The listing builds one solid part. Answer for the finished solid, in the listing's coordinates (mm). Face numbers are marked on the shaded views. Round coordinates to 2 decimals unless told otherwise and drop trailing zeros. Write each loop counter-clockwise with the first axis right and the second up, starting at its lowest first coordinate (ties: lowest second). Pieces come first, ordered by that corner, then holes. Notation, with made-up numbers: M 15.25,-4 L 24.25,-4 A22 cw 24.25,13 Z; hole C 22,-21 d10. An arc over 180 degrees is marked long. Write each question's results on one line, items separated by ' | '.
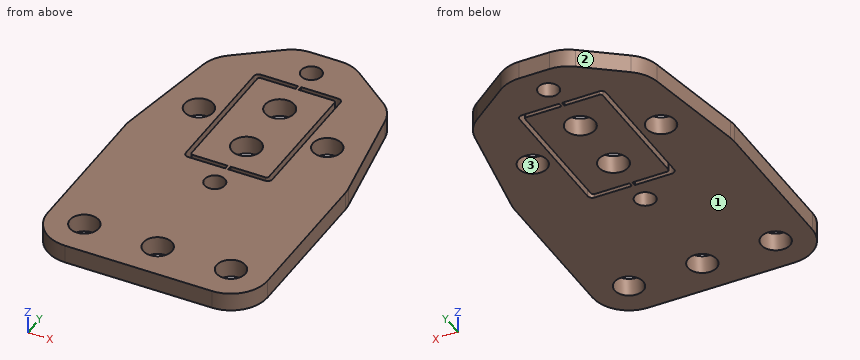
Autodesk Inventor part; units mm, degrees
ref_plane "YZ Plane" through (0, 0, 0) normal (1, 0, 0) x (0, 1, 0)
ref_plane "XZ Plane" through (0, 0, 0) normal (0, 1, 0) x (-1, 0, 0)
ref_plane "XY Plane" through (0, 0, 0) normal (0, 0, 1) x (1, 0, 0)
sketch "Sketch1" plane through (0, 0, 0) normal (0, 0, 1) x (1, 0, 0)
  line L0 (19.05, 12.7) -> (-19.05, 12.7)
  line L1 (-19.05, 12.7) -> (-19.05, -12.7)
  line L2 (-19.05, -12.7) -> (19.05, -12.7)
  line L3 (19.05, -12.7) -> (19.05, 12.7)
  circle A0 centre (-12.7, 0) radius 2.4892
  line L4 (-12.7, 0) -> (12.7, 0)
  circle A1 centre (12.7, 0) radius 2.4892
  line L5 (-19.05, -6.35) -> (19.05, -6.35)
  circle A2 centre (-11.1125, 34.925) radius 2.4892
  line L6 (-11.1125, 34.925) -> (11.1125, 34.925)
  circle A3 centre (11.1125, 34.925) radius 2.4892
  line L7 (-19.05, 12.7) -> (-19.05, 26.343)
  line L8 (-19.05, 26.343) -> (-15.3495, 47.625)
  line L9 (-15.3495, 47.625) -> (15.3495, 47.625)
  line L10 (15.3495, 47.625) -> (19.05, 26.343)
  line L11 (19.05, 26.343) -> (19.05, 12.7)
  circle A4 centre (-11.1125, 34.925) radius 6.35 construction
  circle A5 centre (0, 29.425) radius 2.54
  circle A6 centre (0, 40.425) radius 2.54
  line L12 (0, 40.425) -> (0, 29.425)
  circle A7 centre (0, 0) radius 2.4892
  line L13 (7.493, 46.99) -> (-7.493, 46.99)
  line L14 (-7.493, 46.99) -> (-7.493, 22.86)
  line L15 (-7.493, 22.86) -> (7.493, 22.86)
  line L16 (7.493, 22.86) -> (7.493, 46.99)
  line L17 (7.493, 46.99) -> (-7.493, 22.86) construction
  line L18 (-7.493, 46.99) -> (7.493, 22.86) construction
  circle A8 centre (0, 50.925) radius 1.778
  circle A9 centre (0, 18.925) radius 1.778
  line L19 (-15.3495, 47.625) -> (-4.7625, 55.6875)
  line L20 (4.7625, 55.6875) -> (15.3495, 47.625)
  line L21 (-7.493, 34.925) -> (7.493, 34.925) construction
  line L22 (-7.493, 37.3062) -> (7.493, 37.3062)
  line L23 (-7.493, 34.1313) -> (7.493, 34.1313)
  line L24 (4.7625, 55.6875) -> (-4.7625, 55.6875)
  line L25 (7.493, 37.3062) -> (7.493, 34.1313)
  line L26 (-7.493, 37.3062) -> (-7.493, 34.1313)
  line L27 (-6.6992, 46.1963) -> (6.6992, 46.1963)
  line L28 (6.6992, 46.1963) -> (6.6992, 23.6537)
  line L29 (6.6992, 23.6537) -> (-6.6992, 23.6537)
  line L30 (-6.6992, 23.6537) -> (-6.6992, 46.1963)
  line L31 (0.254, 46.99) -> (-0.254, 46.99)
  line L32 (-0.254, 46.99) -> (-0.254, 46.1963)
  line L33 (-0.254, 46.1963) -> (0.254, 46.1963)
  line L34 (0.254, 46.1963) -> (0.254, 46.99)
  line L35 (0.254, 46.99) -> (-0.254, 46.1963) construction
  line L36 (-0.254, 46.99) -> (0.254, 46.1963) construction
  line L37 (0.254, 22.86) -> (-0.254, 22.86)
  line L38 (-0.254, 22.86) -> (-0.254, 23.6537)
  line L39 (-0.254, 23.6537) -> (0.254, 23.6537)
  line L40 (0.254, 23.6537) -> (0.254, 22.86)
  line L41 (0.254, 22.86) -> (-0.254, 23.6537) construction
  line L42 (-0.254, 22.86) -> (0.254, 23.6537) construction
  point P0 (0, 12.7)
  point P1 (0, 47.625)
  point P2 (0, 34.925)
  point P3 (0, 34.925)
  point P4 (0, 34.925)
  point P5 (-7.493, 34.1313)
  point P6 (7.493, 34.1313)
  point P7 (7.493, 37.3062)
  point P8 (-7.493, 37.3062)
  point P9 (0, 55.6875)
  point P10 (0, -12.7)
  point P11 (0, 46.5931)
  point P12 (0, 46.5931)
  point P13 (0, 23.2569)
  point P14 (0, 23.2569)
  dimension "d0" = 38.1
  dimension "d1" = 25.4
  dimension "d2" = 4.9784
  dimension "d3" = 4.9784
  dimension "d4" = 25.4
  dimension "d5" = 6.35
  dimension "d6" = 4.9784
  dimension "d7" = 22.225
  dimension "d8" = 22.225
  dimension "d9" = 21.282
  dimension "d10" = 12.7
  dimension "d11" = 12.7
  dimension "d12" = 5.08
  dimension "d13" = 11
  dimension "d17" = 24.13
  dimension "d18" = 14.986
  dimension "d19" = 3.556
  dimension "d22" = 360
  dimension "d24" = 32
  dimension "d29" = 0.7937
  dimension "d31" = 3.175
  dimension "d32" = 4.7625
  dimension "d33" = 9.525
  dimension "d51" = 12.7
  dimension "d52" = 6.35
  dimension "d53" = 0.7937
  dimension "d54" = 0.508
extrude "Plate1" add sketch "Sketch1" along normal blind 3.175 contours L3 L5 L1 L0 | L0 L7 L8 L9 L10 L11 | L9 L19 L24 L20 | L30 L22 L12 L6 | L6 L12 L23 L30 | L12 L22 L28 L6 | L6 L28 L23 L12 | L23 L28 L29 L30 | L30 L27 L28 L22 | L13 L34 L27 L32 | L38 L29 L40 L15
fillet "Corner Round2" radius 6.35 8 edges at (19.05, -6.35, 1.5875) (-19.05, -6.35, 1.5875) (19.05, 26.343, 1.5875) (-15.3495, 47.625, 1.5875) (-4.7625, 55.6875, 1.5875) (4.7625, 55.6875, 1.5875) (15.3495, 47.625, 1.5875) (-19.05, 26.343, 1.5875)
cut "Cut1" [suppressed]
fillet "Corner Round3" radius 0.7937 4 edges at (-7.493, 46.99, 1.5875) (-7.493, 22.86, 1.5875) (7.493, 22.86, 1.5875) (7.493, 46.99, 1.5875)
fillet "Corner Round4" radius 0.3969 4 edges at (6.6992, 46.1963, 1.5875) (-6.6992, 46.1963, 1.5875) (-6.6992, 23.6537, 1.5875) (6.6992, 23.6537, 1.5875)
sketch "Sketch4" plane through (0, 0, 3.175) normal (0, 0, 1) x (1, 0, 0)
  line L0 (0.254, 46.99) -> (6.6992, 46.99)
  arc A0 (7.493, 46.1963) -> (6.6992, 46.99) centre (6.6992, 46.1963) ccw
  line L1 (7.493, 46.1963) -> (7.493, 23.6538)
  arc A1 (6.6992, 22.86) -> (7.493, 23.6538) centre (6.6992, 23.6538) ccw
  line L2 (6.6992, 22.86) -> (0.254, 22.86)
  arc A2 (-7.493, 23.6538) -> (-6.6993, 22.86) centre (-6.6993, 23.6538) ccw
  line L3 (-7.493, 23.6538) -> (-7.493, 46.1963)
  arc A3 (-6.6993, 46.99) -> (-7.493, 46.1963) centre (-6.6993, 46.1963) ccw
  arc A4 (-18.9561, 26.8828) -> (-19.05, 25.795) centre (-12.7, 25.795) ccw
  line L4 (-19.05, 0) -> (-19.05, 25.795)
  arc A5 (-19.05, 0) -> (-12.7, -6.35) centre (-12.7, 0) ccw
  line L5 (12.7, -6.35) -> (-12.7, -6.35)
  arc A6 (12.7, -6.35) -> (19.05, 0) centre (12.7, 0) ccw
  line L6 (19.05, 25.795) -> (19.05, 0)
  arc A7 (19.05, 25.795) -> (18.9561, 26.8828) centre (12.7, 25.795) ccw
  line L7 (15.7763, 45.1704) -> (18.9561, 26.8828)
  arc A8 (15.7763, 45.1704) -> (13.3674, 49.1345) centre (9.5202, 44.0826) ccw
  line L8 (6.4671, 54.3894) -> (13.3674, 49.1345)
  arc A9 (6.4671, 54.3894) -> (2.6199, 55.6875) centre (2.6199, 49.3375) ccw
  line L9 (-2.6199, 55.6875) -> (2.6199, 55.6875)
  arc A10 (-2.6199, 55.6875) -> (-6.4671, 54.3894) centre (-2.6199, 49.3375) ccw
  line L10 (-13.3674, 49.1345) -> (-6.4671, 54.3894)
  arc A11 (-13.3674, 49.1345) -> (-15.7763, 45.1704) centre (-9.5202, 44.0826) ccw
  line L11 (-18.9561, 26.8828) -> (-15.7763, 45.1704)
  circle A12 centre (11.1125, 34.925) radius 2.4892
  circle A13 centre (-11.1125, 34.925) radius 2.4892
  circle A14 centre (0, 18.925) radius 1.778
  circle A15 centre (0, 0) radius 2.4892
  circle A16 centre (12.7, 0) radius 2.4892
  circle A17 centre (-12.7, 0) radius 2.4892
  circle A18 centre (0, 50.925) radius 1.778
  line L12 (-27.7407, 9.4742) -> (24.6669, 9.4742)
  arc A19 (-11.4438, 46.6085) -> (-12.6483, 44.6265) centre (-9.5202, 44.0826) ccw
  line L13 (-11.4438, 46.6085) -> (-4.5435, 51.8634)
  arc A20 (-2.6199, 52.5125) -> (-4.5435, 51.8634) centre (-2.6199, 49.3375) ccw
  line L14 (-2.6199, 52.5125) -> (2.6199, 52.5125)
  arc A21 (4.5435, 51.8634) -> (2.6199, 52.5125) centre (2.6199, 49.3375) ccw
  line L15 (4.5435, 51.8634) -> (11.4438, 46.6085)
  arc A22 (12.6483, 44.6265) -> (11.4438, 46.6085) centre (9.5202, 44.0826) ccw
  line L16 (12.6483, 44.6265) -> (15.8281, 26.3389)
  arc A23 (15.875, 25.795) -> (15.8281, 26.3389) centre (12.7, 25.795) ccw
  line L17 (15.875, 25.795) -> (15.875, 0)
  arc A24 (12.7, -3.175) -> (15.875, 0) centre (12.7, 0) ccw
  line L18 (12.7, -3.175) -> (-12.7, -3.175)
  arc A25 (-15.875, 0) -> (-12.7, -3.175) centre (-12.7, 0) ccw
  line L19 (-15.875, 0) -> (-15.875, 25.795)
  arc A26 (-15.8281, 26.3389) -> (-15.875, 25.795) centre (-12.7, 25.795) ccw
  line L20 (-15.8281, 26.3389) -> (-12.6483, 44.6265)
  line L21 (-8.6233, 15.877) -> (8.6233, 15.877)
  line L22 (8.6233, 15.877) -> (15.8281, 26.3389)
  line L23 (-8.6233, 15.877) -> (-15.8281, 26.3389)
  line L24 (-8.6233, 15.877) -> (-8.6233, 5.6134)
  line L25 (-8.6233, 5.6134) -> (-15.875, 5.6134)
  line L26 (8.6233, 15.877) -> (8.6233, 5.6134)
  line L27 (8.6233, 5.6134) -> (15.875, 5.6134)
  line L28 (-10.0711, 17.9793) -> (-10.0711, 5.6134)
  line L29 (10.0711, 17.9793) -> (10.0711, 5.6134)
  arc A27 (6.3024, 23.6537) -> (6.6992, 24.0506) centre (6.3024, 24.0506) ccw
  line L30 (6.6992, 45.7994) -> (6.6992, 24.0506)
  arc A28 (6.6992, 45.7994) -> (6.3024, 46.1963) centre (6.3024, 45.7994) ccw
  line L31 (0.254, 46.1963) -> (6.3024, 46.1963)
  line L32 (0.254, 46.99) -> (0.254, 46.1963)
  line L33 (0.254, 23.6537) -> (0.254, 22.86)
  line L34 (6.3024, 23.6537) -> (0.254, 23.6537)
  arc A29 (-6.6992, 24.0506) -> (-6.3024, 23.6537) centre (-6.3024, 24.0506) ccw
  line L35 (-0.254, 23.6537) -> (-6.3024, 23.6537)
  line L36 (-0.254, 22.86) -> (-0.254, 23.6537)
  line L37 (-0.254, 22.86) -> (-6.6993, 22.86)
  line L38 (-6.6993, 46.99) -> (-0.254, 46.99)
  line L39 (-0.254, 46.1963) -> (-0.254, 46.99)
  line L40 (-6.3024, 46.1963) -> (-0.254, 46.1963)
  arc A30 (-6.3024, 46.1963) -> (-6.6992, 45.7994) centre (-6.3024, 45.7994) ccw
  line L41 (-6.6992, 24.0506) -> (-6.6992, 45.7994)
  point P0 (0, 15.877)
  dimension "d59" = 9.4742
  dimension "d60" = 3.175
  dimension "d61" = 17.2466
  dimension "d62" = 3.048
  dimension "d63" = 1.4478
  dimension "d67" = 5.6134
cut "Cut2" [suppressed]
feature "Corner Round5" [suppressed]
equation "\"d55\" = Thickness"
equation "\"d64\" = Thickness"
equation "\"d35\" = Thickness"
equation "\"BendReliefWidth\" = Thickness"
equation "\"BendReliefDepth\" = 0.5 * Thickness"
equation "\"CornerReliefSize\" = 4 * Thickness"
equation "\"MinimumRemnant\" = 2 * Thickness"
equation "\"TransitionRadius\" = BendRadius"
equation "\"JacobiRadiusSize\" = BendRadius"
equation "\"GapSize\" = Thickness"
properties part number "Standard Sensor Mount" material "Aluminum 6061"
1) Each of these flat-tipped pins is pushed along its axis until it touches: pin 1 (1 mm diameter, centred on y = 48.5, z = 2.5, fed in from +X); pin 2 (1 mm diameter, centred on y = 47, z = 2.5, fed in from +X). Where does it stop, or does it pass through?
Return value:
pin 1: x = 14.52 | pin 2: x = 15.39
2) Section A-A (y = 36.5) is taken. Determine the outline of the cut face in (x, z) (3 decimals).
Return value:
outline: M -17.284,0 L -13.04,0 L -13.04,3.175 L -17.284,3.175 Z; M -9.185,0 L -7.493,0 L -7.493,3.175 L -9.185,3.175 Z; M -6.699,0 L 6.699,0 L 6.699,3.175 L -6.699,3.175 Z; M 7.493,0 L 9.185,0 L 9.185,3.175 L 7.493,3.175 Z; M 13.04,0 L 17.284,0 L 17.284,3.175 L 13.04,3.175 Z
3) Section C-C (z = 0.85) is taken. State how many separate pieces and enclosed holes the cut face has, then the cut area to 3 significant figures.
Return value:
separate pieces: 1 | enclosed holes: 11 | area: 1,900 mm²
4) The mould has two halves that part along X. Classify the marked faces 1, 2 and 3: +X half, -X half, draft (parallel to the pull), parting line (faces both ways), or undercut.
Return value:
face 1: draft | face 2: -X half | face 3: undercut
5) Section B-B (x = 5) is taken. Determine the outline of the cut face in (y, z) (3 decimals).
Return value:
outline: M -6.35,0 L 22.86,0 L 22.86,3.175 L -6.35,3.175 Z; M 23.654,0 L 46.196,0 L 46.196,3.175 L 23.654,3.175 Z; M 46.99,0 L 55.225,0 L 55.225,3.175 L 46.99,3.175 Z
6) Find the intervals of material crossed by line 1 (X direction, y = 25, z = 0.5); line 2 (X direction, y = 34, z = 2); line 3 (Y direction, x = -12.7, z = 1.5), in increasing order.
Return value:
line 1: -19.05 to -7.49, -6.7 to 6.7, 7.49 to 19.05 | line 2: -17.72 to -13.42, -8.8 to -7.49, -6.7 to 6.7, 7.49 to 8.8, 13.42 to 17.72 | line 3: -6.35 to -2.49, 2.49 to 33.01, 36.84 to 49.64
